from build123d import *

# Parameters (mm, degrees)
F1_DEPTH = 15.5
F2_SIZE  = 3
F3_T     = -1.25
F4_DEPTH = 11


with BuildPart() as f1:
    # F0 (on Top) → F1 (new body)
    with BuildSketch(Plane.XY):
        Polygon((9.512444, -7.315286), (11.30742, -4.017743), (11.995546, -0.326916), (11.509465, 3.395912), (9.896757, 6.786325), (7.315286, 9.512444), (4.017743, 11.30742), (0.326916, 11.995546), (-3.395912, 11.509465), (-6.786325, 9.896757), (-9.512444, 7.315286), (-11.30742, 4.017743), (-11.995546, 0.326916), (-11.509465, -3.395912), (-9.896757, -6.786325), (-7.315286, -9.512444), (-4.017743, -11.30742), (-0.326916, -11.995546), (3.395912, -11.509465), (6.786325, -9.896757), align=None)
        with BuildLine():
            ThreePointArc((-3.545, 3.652544), (5.09, 0), (-3.545, -3.652544))
            ThreePointArc((-3.545, -3.652544), (-5.09, 0), (-3.545, 3.652544))
        make_face(mode=Mode.SUBTRACT)
        with BuildLine():
            Line((-3.545, 3.652544), (-3.545, -3.652544))
            ThreePointArc((-3.545, -3.652544), (5.09, 0), (-3.545, 3.652544))
        make_face()
        with BuildLine():
            ThreePointArc((-1.545, 2.676018), (3.09, 0), (-1.545, -2.676018))
            Line((-1.545, -2.676018), (-1.545, 2.676018))
        make_face(mode=Mode.SUBTRACT)
        with BuildLine():
            Line((-1.545, 2.676018), (-1.545, -2.676018))
            ThreePointArc((-1.545, -2.676018), (3.09, 0), (-1.545, 2.676018))
        make_face()
        with BuildLine():
            ThreePointArc((-3.545, 3.652544), (-5.09, 0), (-3.545, -3.652544))
            Line((-3.545, -3.652544), (-3.545, 3.652544))
        make_face()
    extrude(amount=F1_DEPTH)

    # F2
    f2_edges = [f1.edges().sort_by_distance(p)[0] for p in [
        (-10.703111, -5.091118, 0),
        (-8.606021, -8.149385, 0),
        (-5.666514, -10.409932, 0),
        (-2.172329, -11.651483, 0),
        (1.534498, -11.752505, 0),
        (5.091118, -10.703111, 0),
        (8.149385, -8.606021, 0),
        (10.409932, -5.666514, 0),
        (11.651483, -2.172329, 0),
        (11.752505, 1.534498, 0),
        (10.703111, 5.091118, 0),
        (8.606021, 8.149385, 0),
        (5.666514, 10.409932, 0),
        (2.172329, 11.651483, 0),
        (-1.534498, 11.752505, 0),
        (-5.091118, 10.703111, 0),
        (-8.149385, 8.606021, 0),
        (-10.409932, 5.666514, 0),
        (-11.651483, 2.172329, 0),
        (-11.752505, -1.534498, 0),
    ]]
    chamfer(f2_edges, length=F2_SIZE)

    # F3
    f3_openings = [f1.faces().sort_by_distance(p)[0] for p in [
        (0, 0, 15.5),
    ]]
    offset(amount=F3_T, openings=f3_openings)

    # F0 (on Top) → F4 (join)
    with BuildSketch(Plane.XY):
        with BuildLine():
            Line((-3.545, 3.652544), (-3.545, -3.652544))
            ThreePointArc((-3.545, -3.652544), (5.09, 0), (-3.545, 3.652544))
        make_face()
        with BuildLine():
            ThreePointArc((-1.545, 2.676018), (3.09, 0), (-1.545, -2.676018))
            Line((-1.545, -2.676018), (-1.545, 2.676018))
        make_face(mode=Mode.SUBTRACT)
        with BuildLine():
            ThreePointArc((-3.545, 3.652544), (-5.09, 0), (-3.545, -3.652544))
            Line((-3.545, -3.652544), (-3.545, 3.652544))
        make_face()
    extrude(amount=F4_DEPTH)


solid = f1.part
CAD build for the part. Positions are in the model's coordinates, mm. A direction names the side the tool comes from. Give positions to 0.01 mm unless a question says otherwise; leave off trailing zeros. Write each question's results on one line, items separated by ' | '.
Q1. Mould opens along X. For faces 3 (the face through (-9.341, -4.414, 1.479)), 4 (the face through (7.715, 7.273, 9.425)), 5 (the face through (10.7, 5.1, 9.2)), 6 (the face through (4.5, -9.6, 9.4)) say: pulls with the +X half, pulls with the -X half, needs draft (parallel to the pull), parting line crosses it, or undercut.
Geometry check:
face 3: pulls with the -X half | face 4: undercut | face 5: pulls with the +X half | face 6: undercut
Q2. Flat gauge pins, fed straight in: P1, Ø5, axis at x = 2, y = 1, coming from the +Z side; P2, Ø1, axis at y = 0.5, z = 2, coming from the -X side; P3, Ø8, axis at x = 7.5, z = 13, coming from the -Y side. Where does each tip first touch, or does it go through?
Geometry check:
P1: stops at z = 11 | P2: stops at x = -11.46 | P3: stops at y = -11.46
Q3. Which spindle directions (+Z, -Z, +X, -X, +Y, -Y) get a long thin tool onto all of the face, cutting with end or side? Do faces 1 (the face through (-4.414, 9.341, 1.479)), 2 (the face through (-10.516, -1.349, 9.425)). Say none if no direction does.
Geometry check:
face 1: -Z, -X, +Y | face 2: +Z
Q4. Band-saw the part on A-A on z = 8.5. Give the number of separate pieces and of enclosed holes in the cut face, and give its area (3 significant figures).
Geometry check:
separate pieces: 2 | enclosed holes: 2 | area: 146 mm²
Q5. Probe probe 1 along Y at (x, z) = (0, 9); probe 2 along Y at (x, z) = (0.5, 3.5); probe 3 along Z at (x, y) = (0, -2.75). List the from-to ranges inside material, lowest first.
Geometry check:
probe 1: y = -11.95 to -10.69, -5.09 to -3.09, 3.09 to 5.09, 10.69 to 11.95 | probe 2: y = -11.89 to -10.61, -5.07 to -3.05, 3.05 to 5.07, 10.67 to 11.96 | probe 3: z = 0 to 1.25
